Verification items for the finished model (mm, model axes). A direction names the side the tool comes from. Coordinates: 2 decimals unless noted, no trailing zeros. Loops run counter-clockwise (first coordinate to the right, second up) from the corner with the lowest first, then second, coordinate; pieces in that order, holes last. Notation, with made-up numbers: (79.25, -9) -> (117.25, -9) arc R22 ccw to (117.25, 18) -> close; hole circle Ø5 at (47, -22.75). An arc over 180 degrees is marked (long way). Write item = value, one per line.
```python
from build123d import *

# Parameters (mm, degrees)
BOSS_EXTRUDE1_REACH = 17.92
SKETCH3_R           = 2.0335875
FILLET1_R           = 0.24638
CHAMFER1_SIZE       = 0.280736842
CHAMFER1_SIZE2      = 0.07522321


with BuildPart() as part:
    # Sketch2 → Revolve1 (revolve)
    with BuildSketch(Plane.XY, mode=Mode.PRIVATE) as revolve1_sk:
        with BuildLine():
            Line((-7.5819, 0), (7.5819, 0))
            Line((7.5819, 0), (7.5819, 2.0335875))
            Line((7.5819, 2.0335875), (7.08914, 3.25755))
            ThreePointArc((7.08914, 3.25755), (6.10362, 3.429), (5.1181, 3.25755))
            Line((5.1181, 3.25755), (5.1181, 2.003369298))
            ThreePointArc((5.1181, 2.003369298), (5.106940768, 1.97642853), (5.08, 1.965269298))
            ThreePointArc((5.08, 1.965269298), (5.053059232, 1.954110067), (5.0419, 1.927169298))
            Line((5.0419, 1.927169298), (5.0419, 1.261978947))
            Line((5.0419, 1.261978947), (-7.5819, 1.261978947))
            Line((-7.5819, 1.261978947), (-7.5819, 0))
        make_face()
    revolve(revolve1_sk.sketch.rotate(Axis((-7.5819, 0, 0), (-1, 0, 0)), 90), axis=Axis((-7.5819, 0, 0), (-1, 0, 0)))

    # Sketch12 → Cut-Revolve3 (revolve, cut)
    with BuildSketch(Plane.XY, mode=Mode.PRIVATE) as cut_revolve3_sk:
        Polygon((7.5819, 1.6256), (6.58098125, 1.6256), (5.642440652, 0), (7.5819, 0), align=None)
    revolve(cut_revolve3_sk.sketch.rotate(Axis((-7.5819, 0, 0), (1, 0, 0)), 270), axis=Axis((-7.5819, 0, 0), (1, 0, 0)), mode=Mode.SUBTRACT)

    # Boss-Extrude1: up to this cone (the profile starts inside it)
    boss_extrude1_end = Plane(origin=(7.5819, 0, 0), z_dir=(1, 0, 0)).offset(-1.939458348) * Cone(1.732e-06, 41.081996047, 23.718700477, align=(Align.CENTER, Align.CENTER, Align.MIN), mode=Mode.PRIVATE)
    # Sketch3 → Boss-Extrude1 (add, up to the surface)
    with BuildSketch(Plane(origin=(7.5819, 0, 0), x_dir=(0, 0, -1), z_dir=(1, 0, 0)), mode=Mode.PRIVATE) as boss_extrude1_sk1:
        Circle(SKETCH3_R)
        with BuildLine():
            ThreePointArc((1.51222877, -0.182266377), (1.594944844, -0.107324354), (1.6256, 0))
            ThreePointArc((1.6256, 0), (1.594944844, 0.107324354), (1.51222877, 0.182266377))
            ThreePointArc((1.51222877, 0.182266377), (1.055858172, 0.6096), (0.913961698, 1.218495343))
            ThreePointArc((0.913961698, 1.218495343), (0.890418039, 1.327600575), (0.8128, 1.407810896))
            ThreePointArc((0.8128, 1.407810896), (0.704526805, 1.434924929), (0.598267073, 1.40076172))
            ThreePointArc((0.598267073, 1.40076172), (0, 1.2192), (-0.598267073, 1.40076172))
            ThreePointArc((-0.598267073, 1.40076172), (-0.704526805, 1.434924929), (-0.8128, 1.407810896))
            ThreePointArc((-0.8128, 1.407810896), (-0.890418039, 1.327600575), (-0.913961698, 1.218495343))
            ThreePointArc((-0.913961698, 1.218495343), (-1.055858172, 0.6096), (-1.51222877, 0.182266377))
            ThreePointArc((-1.51222877, 0.182266377), (-1.594944844, 0.107324354), (-1.6256, 0))
            ThreePointArc((-1.6256, 0), (-1.594944844, -0.107324354), (-1.51222877, -0.182266377))
            ThreePointArc((-1.51222877, -0.182266377), (-1.055858172, -0.6096), (-0.913961698, -1.218495343))
            ThreePointArc((-0.913961698, -1.218495343), (-0.890418039, -1.327600575), (-0.8128, -1.407810896))
            ThreePointArc((-0.8128, -1.407810896), (-0.704526805, -1.434924929), (-0.598267073, -1.40076172))
            ThreePointArc((-0.598267073, -1.40076172), (0, -1.2192), (0.598267073, -1.40076172))
            ThreePointArc((0.598267073, -1.40076172), (0.704526805, -1.434924929), (0.8128, -1.407810896))
            ThreePointArc((0.8128, -1.407810896), (0.890418039, -1.327600575), (0.913961698, -1.218495343))
            ThreePointArc((0.913961698, -1.218495343), (1.055858172, -0.6096), (1.51222877, -0.182266377))
        make_face(mode=Mode.SUBTRACT)
    boss_extrude1_tool1 = extrude(boss_extrude1_sk1.sketch, amount=-BOSS_EXTRUDE1_REACH, mode=Mode.PRIVATE) & boss_extrude1_end
    add(boss_extrude1_tool1.solids().sort_by_distance((7.5819, 0, 1.976069))[0])

    # Cut-Extrude2 cone 1 section (on through the dimple's axis) → Cut-Extrude2 (revolve, cut)
    with BuildSketch(Plane(origin=(7.5819, 0, 0), x_dir=(0, 0, -1), z_dir=(0, 1, 0))):
        Polygon((0, 0), (1.6256, 0), (0, 0.938540598), align=None)
    revolve(axis=Axis((7.5819, 0, 0), (-1, 0, 0)), mode=Mode.SUBTRACT)

    # Fillet1
    fillet1_edges = [part.edges().sort_by_distance(p)[0] for p in [
        (5.1181, 0, 3.25755),
        (7.08914, 0, 3.25755),
    ]]
    fillet(fillet1_edges, radius=FILLET1_R)

    # Chamfer1
    chamfer1_edges = [part.edges().sort_by_distance(p)[0] for p in [
        (-7.5819, 0, 1.261978947),
    ]]
    chamfer1_side = [part.faces().sort_by_distance(p)[0] for p in [
        (-1.27, 0, 1.261978947),
    ]]
    chamfer(chamfer1_edges, length=CHAMFER1_SIZE, length2=CHAMFER1_SIZE2, reference=chamfer1_side[0])


solid = part.part
```
1) Release check for a two-part mould opening along Y. For faces 1 (the face through (5.79, -0.25, 0.06)), 2 (the face through (-1.22, -1.25, 0.16)), 3 (the face through (5.118, -2, 1)) record: pulls with the +Y half, pulls with the -Y half, needs draft (parallel to the pull), parting line crosses it, or undercut.
Ans:
face_1 = undercut
face_2 = parting line crosses it
face_3 = needs draft
2) Material ranges on line 1 (X direction, y = 0, z = 1.75); line 2 (Y direction, x = 1, z = 0); line 3 (Y direction, x = -1, z = 0.5), recorded low to high.
Ans:
line_1 = 5.04 to 7.58
line_2 = -1.26 to 1.26
line_3 = -1.16 to 1.16
3) Sectioned sample at A-A, the plane x = 1. Record the cut outline in (y, z), plus the area to 3 significant figures.
Ans:
outline = circle Ø2.52 at (0, 0)
area = 5.00 mm2
4) Tool access check on faces 4 (the face through (-7.582, 0, 0)), 5 (the face through (6.94, -0.6, 1.06)). Record the directions out of +Z, -Z, +X, -X, +Y, -Y that give a thin tool (end or side, any length) a straight path to the whole face; none if there is none.
Ans:
face_4 = +Z, -Z, -X, +Y, -Y
face_5 = +X
